Input: part model. Units: mm. Frame: model coordinates. A direction names the side the tool comes from. Coordinates: 2 decimals unless noted, no trailing zeros. Loops run counter-clockwise (first coordinate to the right, second up) from the corner with the lowest first, then second, coordinate; pieces in that order, holes last. Notation, with made-up numbers: (7, 40) - (48, 40) arc R29 ccw to (48, 70) - close; hole circle Ø3 at (-7.75, -28). An arc over 180 degrees is marked (long way). Use a Markdown table: item, result. Add a question column.
1. Section query B-B on z = 0. Return the cut outline in (x, y), then the cut area to 3 significant figures.
2. Section query A-A on y = 49.5. Return the cut outline in (x, z).
3. Contact query for flat-ended pins moving along their axis: P1, Ø3, axis at y = 43, z = -9, coming from the +X side; P2, Ø2.5, axis at x = 9.18, z = 0, coming from the +Y side; P3, Ø2, axis at y = 48, z = -5, coming from the +X side. Output: stop coordinate, or through.
4. Access query for faces 1 (the face through (8.21, 34.86, 0.22)), 2 (the face through (-12.714, 34.858, 9.493)), 3 (the face through (14.434, 35, -5)), 4 (the face through (-6.566, 41, -2)), 5 (the face through (11.427, 34.858, 9.648)). Directions: +Z, -Z, +X, -X, +Y, -Y. A direction counts if a zero-diameter tool reaches every point of the face in a straight line with its end or side. Return the directions, or none.
5. Ray query, L1, parallel to X at y = 35.5, z = 0; L2, parallel to Y at x = -0.25, z = 7.75; L3, parallel to Z at x = -4, y = 40. Return the intervals inside material, ascending. Write a range as [from, to].
6. Section query C-C on x = -3. Return the cut outline in (y, z), then the cut area to 3 significant figures.
7. Draft query along X for faces 6 (the face through (-1.65, 45.296, -0.175)), 7 (the face through (5.434, 41, -2)), 8 (the face through (-1, 32.886, 0)). Return one class per face: released by +X, released by -X, zero draft, split by the parting line, or undercut.
8. Section query D-D on z = 10.25. Return the cut outline in (x, y).
```python
from build123d import *

# Parameters (mm, degrees)
SKETCH1_R             = 8
SKETCH1_R_2           = 5
BOSS_EXTRUDE1_DEPTH   = 12.5
SKETCH1_W             = 30
SKETCH1_H             = 4
BOSS_EXTRUDE1_2_DEPTH = 12.5
BOSS_EXTRUDE2_START   = 7.5
BOSS_EXTRUDE2_DEPTH   = 20
SKETCH2_R             = 1
CUT_EXTRUDE1_DEPTH    = 4
CUT_EXTRUDE2_START    = -26
CUT_EXTRUDE2_DEPTH    = 5


with BuildPart() as part:
    # Sketch1 → Boss-Extrude1 (new, symmetric)
    with BuildSketch(Plane.XY):
        with Locations((-0.566068823, 50.177224178)):
            Circle(SKETCH1_R)
        with Locations((-0.566068823, 50.177224178)):
            Circle(SKETCH1_R_2, mode=Mode.SUBTRACT)
    extrude(amount=BOSS_EXTRUDE1_DEPTH, both=True)



with BuildPart() as body_2:
    # Sketch1 → Boss-Extrude1 2 (new, symmetric)
    with BuildSketch(Plane.XY):
        with Locations((-0.566068823, 34.885721556)):
            Rectangle(SKETCH1_W, SKETCH1_H)
    extrude(amount=BOSS_EXTRUDE1_2_DEPTH, both=True)


with BuildPart() as part_1:
    add(part.part)

    add(body_2.part)  # Boss-Extrude2 merges body 2
    # Sketch1<5> → Boss-Extrude2 (add)
    with BuildSketch(Plane.XY.offset(BOSS_EXTRUDE2_START)):
        with BuildLine():
            Line((-6.566068823, 44.885721556), (-6.566068823, 36.885721556))
            Line((-6.566068823, 36.885721556), (5.433931177, 36.885721556))
            Line((5.433931177, 36.885721556), (5.433931177, 44.885721556))
            ThreePointArc((5.433931177, 44.885721556), (-0.566068823, 42.177224178), (-6.566068823, 44.885721556))
        make_face()
    extrude(amount=-BOSS_EXTRUDE2_DEPTH)

    # Sketch2 → Cut-Extrude1 (cut)
    with BuildSketch(Plane.XZ.offset(-32.885721556)):
        with BuildLine():
            ThreePointArc((-15.566068823, 2.5), (-12.637136635, 9.571067812), (-5.566068823, 12.5))
            Line((-5.566068823, 12.5), (-15.566068823, 12.5))
            Line((-15.566068823, 12.5), (-15.566068823, 2.5))
        make_face()
        with Locations(Location((-10.316068823, 0, 0), (0, 0, 270))):
            Circle(SKETCH2_R)
        with BuildLine():
            Line((14.433931177, 12.5), (4.433931177, 12.5))
            ThreePointArc((4.433931177, 12.5), (11.504998989, 9.571067812), (14.433931177, 2.5))
            Line((14.433931177, 2.5), (14.433931177, 12.5))
        make_face()
        with Locations(Location((9.183931177, 0, 0), (0, 0, 270))):
            Circle(SKETCH2_R)
    extrude(amount=-CUT_EXTRUDE1_DEPTH, mode=Mode.SUBTRACT)

    # Cut-Extrude2: read off the stored shape, not the designer's step
    # Cut-Extrude2 outline → Cut-Extrude2 (cut)
    with BuildSketch(Plane.XZ.offset(-32.885721556).offset(CUT_EXTRUDE2_START)):
        with BuildLine():
            add(Edge.make_bspline(
                [(-0.566068823, -4.5), (-0.035293393, -4.5), (0.481128127, -4.281375894), (1.215722466, -3.546490005), (1.433600027, -3.025317772), (1.434261529, -1.977206776), (1.218792073, -1.456508795), (0.477783673, -0.715350376), (-0.041929223, -0.500221589), (-1.08851599, -0.499778769), (-1.610163203, -0.716198326), (-2.348367378, -1.45334182), (-2.565791182, -1.971191938), (-2.566345912, -3.026705842), (-2.348095204, -3.545904648), (-1.614377567, -4.28061319), (-1.096844254, -4.5), (-0.566068823, -4.5)],
                knots=[0, 0, 0, 0, 0.125, 0.125, 0.25, 0.25, 0.375, 0.375, 0.5, 0.5, 0.625, 0.625, 0.75, 0.75, 0.875, 0.875, 1, 1, 1, 1], degree=3))
        make_face()
    extrude(amount=CUT_EXTRUDE2_DEPTH, mode=Mode.SUBTRACT)


solid = part_1.part
```
Resolved:
| question | item | result |
|---|---|---|
| 1 | outline | (-15.57, 32.89) - (-11.32, 32.89) - (-11.32, 36.89) - (-15.57, 36.89) - close; (-9.32, 32.89) - (8.18, 32.89) - (8.18, 36.89) - (5.43, 36.89) - (5.43, 44.89) arc R8 ccw (long way) to (-6.57, 44.89) - (-6.57, 36.89) - (-9.32, 36.89) - close; (10.18, 32.89) - (14.43, 32.89) - (14.43, 36.89) - (10.18, 36.89) - close; hole circle Ø10 at (-0.57, 50.18) |
| 1 | area | 300 mm² |
| 2 | outline | (-8.54, -12.5) - (-5.52, -12.5) - (-5.52, 12.5) - (-8.54, 12.5) - close; (4.39, -12.5) - (7.41, -12.5) - (7.41, 12.5) - (4.39, 12.5) - close |
| 3 | P1 | x = 5.43 |
| 3 | P2 | y = 36.89 |
| 3 | P3 | x = 7.35 |
| 4 | face 1 | +Y, -Y |
| 4 | face 2 | +Z, -X, -Y |
| 4 | face 3 | +Z, -Z, +X, +Y, -Y |
| 4 | face 4 | +Z, -Z, -X |
| 4 | face 5 | +Z, +X, -Y |
| 5 | L1 | [-15.57, -11.32], [-9.32, 8.18], [10.18, 14.43] |
| 5 | L2 | [32.89, 36.89], [42.18, 45.19], [55.17, 58.17] |
| 5 | L3 | [-12.5, 7.5] |
| 6 | outline | (32.89, -12.5) - (45.81, -12.5) - (45.81, 12.5) - (42.56, 12.5) - (42.56, 7.5) - (36.89, 7.5) - (36.89, 12.5) - (32.89, 12.5) - close; (54.54, -12.5) - (57.8, -12.5) - (57.8, 12.5) - (54.54, 12.5) - close |
| 6 | area | 376 mm² |
| 7 | face 6 | undercut |
| 7 | face 7 | released by +X |
| 7 | face 8 | zero draft |
| 8 | outline | (-11.89, 32.89) - (10.75, 32.89) - (10.75, 36.89) - (-11.89, 36.89) - close; circle Ø16 at (-0.57, 50.18); hole circle Ø10 at (-0.57, 50.18) |
